Read the model definition and answer for the solid it produces. Units are mm, in the model's axes. A direction names the side the tool comes from. Give positions to 0.01 mm unless a question says otherwise; leave off trailing zeros. Write each loop counter-clockwise with the first axis right and the second up, starting at its lowest first coordinate (ties: lowest second). Pieces come first, ordered by that corner, then holes. Notation, with made-up numbers: (85, 70) -> (106, 70) arc R19 cw to (106, 106) -> close; hole circle Ø5 at (25.25, 49). An arc over 180 degrees is marked (long way). Put each result on its own line as item: value. Start each with the question number.
from build123d import *

# Parameters (mm, degrees)
SKETCH1_R           = 5
BOSS_EXTRUDE1_DEPTH = 10
CUT_EXTRUDE1_DEPTH  = 8
CHAMFER1_SIZE       = 0.5


with BuildPart() as part:
    # Sketch1 → Boss-Extrude1 (new body)
    with BuildSketch(Plane(origin=(0, 0, 0), x_dir=(1, 0, 0), z_dir=(0, 1, 0))):
        with Locations(Location((0, 0, 0), (0, 0, 270))):
            Circle(SKETCH1_R)
    extrude(amount=BOSS_EXTRUDE1_DEPTH)

    # Sketch2 → Cut-Extrude1 (cut)
    with BuildSketch(Plane(origin=(0, 10, 0), x_dir=(1, 0, 0), z_dir=(0, 1, 0))):
        with BuildLine():
            Line((-1.79933321, 2.555), (1.79933321, 2.555))
            ThreePointArc((1.79933321, 2.555), (0, -3.125), (-1.79933321, 2.555))
        make_face()
    extrude(amount=-CUT_EXTRUDE1_DEPTH, mode=Mode.SUBTRACT)

    # Chamfer1
    chamfer1_edges = [part.edges().sort_by_distance(p)[0] for p in [
        (0, 10, 3.125),
        (0, 10, -2.555),
    ]]
    chamfer(chamfer1_edges, length=CHAMFER1_SIZE)


solid = part.part
1) A cutting plane is placed at A-A on x = 0. Give the vertices of the cut face in (y, z) (3 decimals).
2) A cutting plane is placed at C-C on y = 8.25. Give the vertices of the cut face in (x, z) (3 decimals), and give its area (3 significant figures).
3) For a pull along X with two mould halves and no side action, classify faces 3 (the face through (0, 6, -2.555)), 4 (the face through (-4.88, 4.93, -1.08)), 5 (the face through (0.1, 10, -3.4)) as pulls with the +X half, pulls with the -X half, needs draft (parallel to the pull), parting line crosses it, or undercut.
4) A cutting plane is placed at D-D on y = 1. Give the vertices of the cut face in (x, z), and give its area (3 significant figures).
5) For faces 1 (the face through (0, 0, 0)), 2 (the face through (0.111, 5.802, 3.123)), determine the directions among +Z, -Z, +X, -X, +Y, -Y from which every point of the face is accessible in a straight line to the end or side of a thin tool.
6) A cutting plane is placed at B-B on z = 0. Give the vertices of the cut face in (x, y) (3 decimals).
7) Each of these flat-tipped pins is pushed along its axis until it touches: pin 1 Ø1.1 at (x, y) = (-1, 5.5) entering from +Z; pin 2 Ø1 at (x, y) = (-2.5, 7) entering from +Z; pin 3 Ø6 at (x, z) = (0, 0.5) entering from +Y (3 decimals). Where does it stop, or does it pass through?
8) Straight lines are drawn through the part: line 1 (X direction, y = 7.5, z = 0) (3 decimals); line 2 (Y direction, x = 2, z = 0.75); line 3 (Z direction, x = -0.5, y = 4.5) (3 decimals). For each, find the intervals that lie inside material, in ascending order. Write a range as [from, to].
Results found:
1. outline: (0, -5) -> (10, -5) -> (10, -3.055) -> (9.5, -2.555) -> (2, -2.555) -> (2, 3.125) -> (9.5, 3.125) -> (10, 3.625) -> (10, 5) -> (0, 5) -> close
2. outline: circle Ø10 at (0, 0); hole (-1.799, -2.555) -> (1.799, -2.555) arc R3.125 ccw (long way) to start
2. area: 49.3 mm²
3. face 3: undercut
3. face 4: parting line crosses it
3. face 5: needs draft
4. outline: circle Ø10 at (0, 0)
4. area: 78.5 mm²
5. face 1: +Z, -Z, +X, -X, -Y
5. face 2: +Y
6. outline: (-5, 0) -> (5, 0) -> (5, 10) -> (3.625, 10) -> (3.125, 9.5) -> (3.125, 2) -> (-3.125, 2) -> (-3.125, 9.5) -> (-3.625, 10) -> (-5, 10) -> close
7. pin 1: stops at z = 4.98
7. pin 2: stops at z = 4.58
7. pin 3: stops at y = 9.875
8. line 1: x = [-5, -3.125], [3.125, 5]
8. line 2: y = [0, 2]
8. line 3: z = [-4.975, -2.555], [3.085, 4.975]
